Work out the finished part from the listing and answer in its coordinate system (mm). A direction names the side the tool comes from. Coordinates: 2 decimals unless noted, no trailing zeros. Loops run counter-clockwise (first coordinate to the right, second up) from the corner with the lowest first, then second, coordinate; pieces in that order, holes last. Notation, with made-up numbers: (-34.75, 68.5) -> (-28.75, 68.5) arc R33 cw to (-28.75, 97.5) -> close; hole circle Ø6 at (61, 68). An arc over 180 degrees is marked (long way). One line per question, with ' | ' between items.
```python
from build123d import *

# Parameters (mm, degrees)
F0_R      = 1.65
F0_W      = 165
F0_H      = 100
F1_DEPTH  = 1.7
F2_DEPTH  = 7.45
F3_W      = 157
F3_H      = 89.75
F4_DEPTH  = 0.2
F5_W      = 5
F5_H      = 51.16
F6_DEPTH  = 11.4
F5_W_2    = 26.4
F5_H_2    = 17
F7_DEPTH  = 3
F8_W      = 65.32
F8_H      = 73
F8_R      = 1.6
F8_W_2    = 5
F8_H_2    = 51.16
F9_DEPTH  = 1.2
F11_DEPTH = 6
F10_R     = 6.08
F10_R_2   = 1
F12_DEPTH = 7.85
F10_W     = 9
F10_H     = 20.3
F13_DEPTH = 9.25
F10_R_3   = 1.5
F14_DEPTH = 3.15
F10_W_2   = 6.25
F10_H_2   = 6.25
F15_DEPTH = 2
F10_W_3   = 1.2
F10_H_3   = 7.5
F10_W_4   = 4.5
F16_DEPTH = 2.9


with BuildPart() as f1:
    # F0 (on Top) → F1 (new body)
    with BuildSketch(Plane.XY):
        with BuildLine():
            Line((-87.5, -54), (87.5, -54))
            ThreePointArc((87.5, -54), (89.6213203436, -53.1213203436), (90.5, -51))
            Line((90.5, -51), (90.5, 51))
            ThreePointArc((90.5, 51), (89.6213203436, 53.1213203436), (87.5, 54))
            Line((87.5, 54), (-87.5, 54))
            ThreePointArc((-87.5, 54), (-89.6213203436, 53.1213203436), (-90.5, 51))
            Line((-90.5, 51), (-90.5, -51))
            ThreePointArc((-90.5, -51), (-89.6213203436, -53.1213203436), (-87.5, -54))
        make_face()
        with Locations((-87.5, -51)):
            Circle(F0_R, mode=Mode.SUBTRACT)
        with Locations((87.5, -51)):
            Circle(F0_R, mode=Mode.SUBTRACT)
        with Locations((-87.5, 51)):
            Circle(F0_R, mode=Mode.SUBTRACT)
        Rectangle(F0_W, F0_H, mode=Mode.SUBTRACT)
        with Locations((87.5, 51)):
            Circle(F0_R, mode=Mode.SUBTRACT)
        Rectangle(F0_W, F0_H)
    extrude(amount=-F1_DEPTH)

    # F0 (on Top) → F2 (join)
    with BuildSketch(Plane.XY):
        Rectangle(F0_W, F0_H)
    extrude(amount=F2_DEPTH)

    # F3 (on face) → F4 (cut)
    with BuildSketch(Plane.XY.offset(7.45)):
        with Locations((-1, 2.125)):
            Rectangle(F3_W, F3_H)
    extrude(amount=-F4_DEPTH, mode=Mode.SUBTRACT)

    # F5 (on face) → F6 (join)
    with BuildSketch(Plane(origin=(0, 0, -1.7), x_dir=(1, 0, 0), z_dir=(0, 0, -1))):
        with Locations((86.5, -0.02)):
            Rectangle(F5_W, F5_H)
    extrude(amount=F6_DEPTH)

    # F5 (on face) → F7 (join)
    with BuildSketch(Plane(origin=(0, 0, -1.7), x_dir=(1, 0, 0), z_dir=(0, 0, -1))):
        with Locations((-67, 41.5)):
            Rectangle(F5_W_2, F5_H_2)
    extrude(amount=F7_DEPTH)

    # F8 (on face) → F9 (join)
    with BuildSketch(Plane(origin=(0, 0, -13.1), x_dir=(1, 0, 0), z_dir=(0, 0, -1))):
        with Locations((74.16, 0.1)):
            Rectangle(F8_W, F8_H)
        with Locations((46.5, -31.4)):
            Circle(F8_R, mode=Mode.SUBTRACT)
        with Locations((86.5, -0.02)):
            Rectangle(F8_W_2, F8_H_2, mode=Mode.SUBTRACT)
        with Locations((97.42, -1.15)):
            Circle(F8_R, mode=Mode.SUBTRACT)
        with Locations((46.5, 31.6)):
            Circle(F8_R, mode=Mode.SUBTRACT)
        with Locations((86.5, -0.02)):
            Rectangle(F8_W_2, F8_H_2)
    extrude(amount=F9_DEPTH)

    # F10 (on face) → F11 (join)
    with BuildSketch(Plane.XY.offset(-13.1)):
        Polygon((89, -25.56), (87.19, -25.56), (87.19, -35.79), (98.82, -35.79), (98.82, -25.56), align=None)
    extrude(amount=F11_DEPTH)

    # F10 (on face) → F12 (join)
    with BuildSketch(Plane.XY.offset(-13.1)):
        with Locations((98.6, -10.24)):
            Circle(F10_R)
        with Locations((98.6, -10.24)):
            Circle(F10_R_2, mode=Mode.SUBTRACT)
    extrude(amount=F12_DEPTH)

    # F10 (on face) → F13 (join)
    with BuildSketch(Plane.XY.offset(-13.1)):
        with Locations((99.42, 16.6)):
            Rectangle(F10_W, F10_H)
    extrude(amount=F13_DEPTH)

    # F10 (on face) → F14 (join)
    with BuildSketch(Plane.XY.offset(-13.1)):
        with Locations((94.325, 31.025)):
            Circle(F10_R_3)
        with Locations((99.045, -19.875)):
            Circle(F10_R_3)
    extrude(amount=F14_DEPTH)

    # F10 (on face) → F15 (join)
    with BuildSketch(Plane.XY.offset(-13.1)):
        with Locations((94.325, 31.025)):
            Rectangle(F10_W_2, F10_H_2)
        with Locations((94.325, 31.025)):
            Circle(F10_R_3, mode=Mode.SUBTRACT)
        with Locations((99.045, -19.875)):
            Rectangle(F10_W_2, F10_H_2)
        with Locations((99.045, -19.875)):
            Circle(F10_R_3, mode=Mode.SUBTRACT)
    extrude(amount=F15_DEPTH)

    # F10 (on face) → F16 (join)
    with BuildSketch(Plane.XY.offset(-13.1)):
        with Locations((107.42, 31.65)):
            Rectangle(F10_W_3, F10_H_3)
        with Locations((104.57, 31.65)):
            Rectangle(F10_W_4, F10_H_3)
    extrude(amount=F16_DEPTH)


solid = f1.part
```
1) Find section C-C (x = 18.5). Write down the section's boundary in (y, z), plus the area to 3 significant figures.
Check values:
outline: (-54, -1.7) -> (54, -1.7) -> (54, 0) -> (50, 0) -> (50, 7.45) -> (47, 7.45) -> (47, 7.25) -> (-42.75, 7.25) -> (-42.75, 7.45) -> (-50, 7.45) -> (-50, 0) -> (-54, 0) -> close | area: 911 mm^2
2) Find the intervals of material crossed by line 1 along Y through (x, z) = (-87.5, -0.35); line 2 along Y through (x, z) = (98.6, -8.75); line 3 along X through (y, z) = (-31.6, -13.8), in increasing order.
Check values:
line 1: y = -54 to -52.65, -49.35 to 49.35, 52.65 to 54 | line 2: y = -35.79 to -25.56, -16.32 to -11.24, -9.24 to -4.16, 6.45 to 26.75 | line 3: x = 41.5 to 44.9, 48.1 to 106.82
3) Flat-ended cylindrical pins translate along their axes: pin 1 (3.5 mm diameter, centred on x = 94.5, y = 30.5, fed in from +Z); pin 2 (6 mm diameter, centred on x = -7.5, z = 2.5, fed in from -Y); pin 3 (4 mm diameter, centred on x = 73.5, y = 32.5, fed in from +Z); pin 4 (6.5 mm diameter, centred on y = -31, z = -10, fed in from -X). Find the tip coordinate at first contact, or state that the pin passes through.
Check values:
pin 1: stops at z = -9.95 | pin 2: stops at y = -54 | pin 3: stops at z = 7.25 | pin 4: stops at x = 41.5
4) Find section A-A (x = 70.5). Write down the section's boundary in (y, z), plus the area to 3 significant figures.
Check values:
outline: (-54, -1.7) -> (54, -1.7) -> (54, 0) -> (50, 0) -> (50, 7.45) -> (47, 7.45) -> (47, 7.25) -> (-42.75, 7.25) -> (-42.75, 7.45) -> (-50, 7.45) -> (-50, 0) -> (-54, 0) -> close; (-36.6, -14.3) -> (36.4, -14.3) -> (36.4, -13.1) -> (-36.6, -13.1) -> close | area: 998 mm^2
5) The mould has two halves that part along Y. Classify faces 1 (the face through (94.92, 16, -9)), 2 (the face through (74, -1, -14.3)), 3 (the face through (86, 25.6, -7)): released by +Y, released by -Y, zero draft, split by the parting line, or undercut.
Check values:
face 1: undercut | face 2: zero draft | face 3: released by +Y
6) Find section D-D (y = -38.5). Write down the section's boundary in (x, z).
Check values:
outline: (-90.5, -1.7) -> (-80.2, -1.7) -> (-80.2, -4.7) -> (-53.8, -4.7) -> (-53.8, -1.7) -> (90.5, -1.7) -> (90.5, 0) -> (82.5, 0) -> (82.5, 7.45) -> (77.5, 7.45) -> (77.5, 7.25) -> (-79.5, 7.25) -> (-79.5, 7.45) -> (-82.5, 7.45) -> (-82.5, 0) -> (-90.5, 0) -> close
7) For faces 4 (the face through (99, 26.75, -9)), 5 (the face through (98, -18, -11.1)), 6 (the face through (89, 0, -7)), 7 (the face through (99, 6.45, -9)), 8 (the face through (84, 0, -7)), determine the directions among +Z, -Z, +X, -X, +Y, -Y from which every point of the face is accessible in a straight line to the end or side of a thin tool.
Check values:
face 4: +Z, +X, -X | face 5: +Z | face 6: +Y | face 7: +Z, +X | face 8: -X, +Y, -Y
8) Find section B-B (y = 20.5). Write down the section's boundary in (x, z), plus the area to 3 significant figures.
Check values:
outline: (-90.5, -1.7) -> (84, -1.7) -> (84, -13.1) -> (41.5, -13.1) -> (41.5, -14.3) -> (106.82, -14.3) -> (106.82, -13.1) -> (103.92, -13.1) -> (103.92, -3.85) -> (94.92, -3.85) -> (94.92, -13.1) -> (89, -13.1) -> (89, -1.7) -> (90.5, -1.7) -> (90.5, 0) -> (82.5, 0) -> (82.5, 7.45) -> (77.5, 7.45) -> (77.5, 7.25) -> (-79.5, 7.25) -> (-79.5, 7.45) -> (-82.5, 7.45) -> (-82.5, 0) -> (-90.5, 0) -> close | area: 1,720 mm^2
